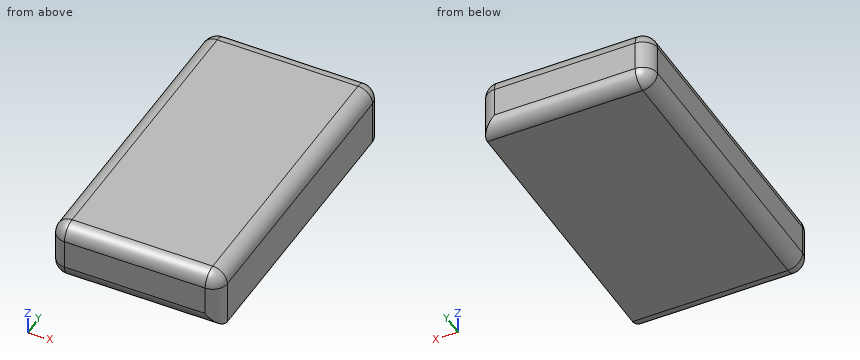
Autodesk Fusion 360 part; units mm, degrees
sketch "Sketch1" plane through (0, 0, 0) normal (0, 0, 1) x (1, 0, 0)
  line L0 (-14.5, 26.5) -> (14.5, 26.5)
  line L1 (14.5, 26.5) -> (14.5, -26.5)
  line L2 (14.5, -26.5) -> (-14.5, -26.5)
  line L3 (-14.5, -26.5) -> (-14.5, 26.5)
  dimension "d1" = 29
  dimension "d2" = 53
extrude "Extrude1" add sketch "Sketch1" along normal blind 10
fillet "Fillet1" radius 2.5 9 edges at (-14.5, -26.5, 5) (0, 26.5, 10) (-14.5, 26.5, 5) (0, 26.5, 0) (14.5, 0, 10) (0, -26.5, 10) (-14.5, 0, 0) (-14.5, 0, 10) (14.5, 26.5, 5) 4 faces at (4.8333, -26.5, 3.3333) (-4.8333, 26.5, 3.3333) (-4.8333, -8.8333, 10) (-14.5, -8.8333, 3.3333)
Verification items for the finished model (mm, model axes). Coordinates: 2 decimals unless noted, no trailing zeros. Order: outer loops, then holes, each group sorted by start corner. A loop starts at its lowest first (then second) coordinate and runs counter-clockwise, first axis right, second up. Notation, with made-up numbers: M 28,-24.5 L 85,-24.5 A12 ccw 85,-12.5 Z; hole C 67.5,77 d8. An arc over 180 degrees is marked long. Write each question's results on one line, items separated by ' | '.
1) Scan lines: line 1 along Y through (x, z) = (-1.75, 2.25); line 2 along X through (y, z) = (15, 7.75); line 3 along Y through (x, z) = (-9.5, 9). Record each from-to range of solid material in increasing order. Write a range as [from, to].
Solved:
line 1: y = [-26.49, 26.49] | line 2: x = [-14.49, 14.49] | line 3: y = [-26, 26]
2) Section check B-B on z = 1.5. Record the cut outline in (x, y).
Solved:
outline: M -14.29,-24 A2.29 ccw -12,-26.29 L 13,-26.29 A2.5 ccw 14.5,-24 L 14.5,24 A2.5 ccw 13,26.29 L -12,26.29 A2.29 ccw -14.29,24 Z
3) Section check A-A on z = 9. Record the cut outline in (x, y), plus the area to 3 significant figures.
Solved:
outline: M -14,-24 A2 ccw -12,-26 L 12,-26 A2 ccw 14,-24 L 14,24 A2 ccw 12,26 L -12,26 A2 ccw -14,24 Z | area: 1,450 mm²
4) Gauge pin test, flat end, axial feed: pin 1 Ø1 at (x, z) = (-10, 1.5) entering from +Y. Record the tip position at first contact, or that the pin passes through.
Solved:
pin 1: stops at y = 26.45
